Model file for the job. Use its own axes, mm. A direction names the side the tool comes from. Round coordinates to 2 decimals unless told otherwise and drop trailing zeros. Loops run counter-clockwise (first coordinate to the right, second up) from the corner with the lowest first, then second, coordinate; pieces in that order, holes last. Notation, with made-up numbers: M 79.5,-34.75 L 133.5,-34.75 A9 ccw 133.5,-19.75 Z; hole C 18,51 d9. An arc over 180 degrees is marked long. Use a Markdown table: item, result. Add a question column.
Q1. Mould opens along X. For faces 1 (the face through (-1.859, 1.797, 19.72)), 2 (the face through (-51, -41, 133.971)), 3 (the face through (5, 3, 20)) say: +X half, -X half, draft (parallel to the pull), parting line (faces both ways), or undercut.
Q2. Probe line 1 (Z direction, x = 5.5, y = 2.3); line 2 (Y direction, x = 2, z = 22); line 3 (X direction, y = 1, z = 10). List the from-to ranges inside material, lowest first. Write a range as from..to.
Q3. Tool access for faces 4 (the face through (-1, -25, 16)), 5 (the face through (-87.05, -41.056, 113.966)), 6 (the face through (-1, -9, 40)), 7 (the face through (-3, -23, 36)), 8 (the face through (0, -23, 36)): list every direction of +Z, -Z, +X, -X, +Y, -Y with a clear straight run to the whole face (end or side of a thin tool).
Q4. Cut at B-B (x = -54.5). Give the cut face in (y, z).
Q5. Pin check, flat tips, straight feed: pin 1 (3 mm diameter, centred on x = 5.5, z = 10, fed in from -Y); pin 2 (22 mm diameter, centred on y = -24.5, z = 51.5, fed in from +X); pin 3 (1.5 mm diameter, centred on x = -1, z = 16.5, fed in from -Y). Stop position of each tip, or through.
Q6. Cut at C-C (y = -8). Give the cut face in (x, z), plus the area to 3 significant figures.
Q7. Cut at A-A (z = 105). Give the cut face in (x, y), plus the area to 3 significant figures.
from build123d import *

# Parameters (mm, degrees)
SM_BASE_FLANGE_1_DEPTH           = 40
M3X0_5_1_D                       = 2.5
SKETCH_22_W                      = 3
SKETCH_22_H                      = 12
EXTRUDE_6_DEPTH                  = 12
SKETCH_23_W                      = 3
SKETCH_23_H                      = 67
EXTRUDE_7_DEPTH                  = 8
CHAMFER_1_SIZE                   = 10
CHAMFER_2_SIZE                   = 5
SM_EDGE_FLANGE_1_STRIP_CUT_DEPTH = 8
SM_EDGE_FLANGE_1_DEPTH           = 8
SM_EDGE_FLANGE_2_STRIP_CUT_DEPTH = 8
SM_EDGE_FLANGE_2_DEPTH           = 8
SM_EDGE_FLANGE_3_STRIP_CUT_DEPTH = 8
SM_EDGE_FLANGE_3_DEPTH           = 8


# Sheet-metal steps are written as plain solids
with BuildPart() as part:
    # 草圖3 → 基材-凸緣1 (new body)
    with BuildSketch(Plane.XY):
        with BuildLine():
            Line((10, 0), (1, 0))
            ThreePointArc((1, 0), (0.292893219, -0.292893219), (0, -1))
            Line((0, -1), (0, -25))
            Line((0, -25), (-3, -25))
            Line((-3, -25), (-3, -1))
            ThreePointArc((-3, -1), (-1.828427125, 1.828427125), (1, 3))
            Line((1, 3), (10, 3))
            Line((10, 3), (10, 0))
        make_face()
    extrude(amount=SM_BASE_FLANGE_1_DEPTH)

    # M3x0.5 螺紋孔1 (through all)
    with Locations(Plane(origin=(0, 3, 0), x_dir=(1, 0, 0), z_dir=(0, 1, 0))):
        with Locations((5.5, -30), (5.5, -10)):
            Hole(M3X0_5_1_D / 2)

    # 草圖22 → 填料-伸長6 (add)
    with BuildSketch(Plane.XZ.offset(25)):
        with Locations((-1.5, 34)):
            Rectangle(SKETCH_22_W, SKETCH_22_H)
    extrude(amount=EXTRUDE_6_DEPTH)

    # 草圖23 → 填料-伸長7 (add)
    with BuildSketch(Plane.XZ.offset(37)):
        with Locations((-1.5, 61.5)):
            Rectangle(SKETCH_23_W, SKETCH_23_H)
    extrude(amount=EXTRUDE_7_DEPTH)

    # 導角1
    chamfer_1_edges = [part.edges().sort_by_distance(p)[0] for p in [
        (-1.5, -37, 40),
        (-1.5, -45, 28),
    ]]
    chamfer(chamfer_1_edges, length=CHAMFER_1_SIZE)

    # 導角2
    chamfer_2_edges = [part.edges().sort_by_distance(p)[0] for p in [
        (-1.5, -25, 0),
    ]]
    chamfer(chamfer_2_edges, length=CHAMFER_2_SIZE)

    # 邊線-凸緣1 strip (across the edge) → 邊線-凸緣1 strip cut (cut)
    with BuildSketch(Plane(origin=(-3, -45, 95), x_dir=(-0.8660254037844416, 0, -0.49999999999999495), z_dir=(0, 1, 0))):
        Polygon((-9.464101615, 10.392304845), (-2.464101615, -1.732050808), (0.133974596, -0.232050808), (-6.866025404, 11.892304845), align=None)
    extrude(amount=SM_EDGE_FLANGE_1_STRIP_CUT_DEPTH, mode=Mode.SUBTRACT)

    # 邊線-凸緣1 section (across the edge) → 邊線-凸緣1 (add)
    with BuildSketch(Plane(origin=(-3, -45, 95), x_dir=(-0.8660254037844416, 0, -0.49999999999999495), z_dir=(0, 1, 0))):
        with BuildLine():
            Line((-3, 0.267949192), (-3, 45))
            Line((-3, 45), (0, 45))
            Line((0, 45), (0, 0.267949192))
            ThreePointArc((0, 0.267949192), (0.034074174, 0.009130147), (0.133974596, -0.232050808))
            Line((0.133974596, -0.232050808), (-2.464101615, -1.732050808))
            ThreePointArc((-2.464101615, -1.732050808), (-2.863703305, -0.767326988), (-3, 0.267949192))
        make_face()
    extrude(amount=SM_EDGE_FLANGE_1_DEPTH)

    # 邊線-凸緣2 strip (across the edge) → 邊線-凸緣2 strip cut (cut)
    with BuildSketch(Plane(origin=(-25.5, -45, 133.97114317), x_dir=(0, 0, -1), z_dir=(0, 1, 0))):
        Polygon((-13.124355653, 4.113248654), (-1, -2.886751346), (0.5, -0.288675135), (-11.624355653, 6.711324865), align=None)
    extrude(amount=SM_EDGE_FLANGE_2_STRIP_CUT_DEPTH, mode=Mode.SUBTRACT)

    # 邊線-凸緣2 section (across the edge) → 邊線-凸緣2 (add)
    with BuildSketch(Plane(origin=(-25.5, -45, 133.97114317), x_dir=(0, 0, -1), z_dir=(0, 1, 0))):
        with BuildLine():
            Line((-3, 0.577350269), (-3, 50))
            Line((-3, 50), (0, 50))
            Line((0, 50), (0, 0.577350269))
            ThreePointArc((0, 0.577350269), (0.133974596, 0.077350269), (0.5, -0.288675135))
            Line((0.5, -0.288675135), (-1, -2.886751346))
            ThreePointArc((-1, -2.886751346), (-2.464101615, -1.422649731), (-3, 0.577350269))
        make_face()
    extrude(amount=SM_EDGE_FLANGE_2_DEPTH)

    # 邊線-凸緣3 strip (across the edge) → 邊線-凸緣3 strip cut (cut)
    with BuildSketch(Plane(origin=(-75.5, -45, 133.97114317), x_dir=(0.8660254037844312, 0, -0.5000000000000132), z_dir=(0, 1, 0))):
        Polygon((-13.124355653, 4.113248654), (-1, -2.886751346), (0.5, -0.288675135), (-11.624355653, 6.711324865), align=None)
    extrude(amount=SM_EDGE_FLANGE_3_STRIP_CUT_DEPTH, mode=Mode.SUBTRACT)

    # 邊線-凸緣3 section (across the edge) → 邊線-凸緣3 (add)
    with BuildSketch(Plane(origin=(-75.5, -45, 133.97114317), x_dir=(0.8660254037844312, 0, -0.5000000000000132), z_dir=(0, 1, 0))):
        with BuildLine():
            Line((-3, 0.577350269), (-3, 45))
            Line((-3, 45), (0, 45))
            Line((0, 45), (0, 0.577350269))
            ThreePointArc((0, 0.577350269), (0.133974596, 0.077350269), (0.5, -0.288675135))
            Line((0.5, -0.288675135), (-1, -2.886751346))
            ThreePointArc((-1, -2.886751346), (-2.464101615, -1.422649731), (-3, 0.577350269))
        make_face()
    extrude(amount=SM_EDGE_FLANGE_3_DEPTH)


solid = part.part
Checked values:
| question | item | result |
|---|---|---|
| 1 | face 1 | -X half |
| 1 | face 2 | undercut |
| 1 | face 3 | draft |
| 2 | line 1 | z = 0..8.75, 11.25..28.75, 31.25..40 |
| 2 | line 2 | y = 0..3 |
| 2 | line 3 | x = -2.46..4.25, 6.75..10 |
| 3 | face 4 | -Z, +X, -X, -Y |
| 3 | face 5 | -Z, +Y, -Y |
| 3 | face 6 | +Z, +X, -X, +Y |
| 3 | face 7 | -Z, -X, +Y, -Y |
| 3 | face 8 | +Z, -Z, +X, -Y |
| 4 | outline | M -45,133.97 L -37,133.97 L -37,136.97 L -45,136.97 Z |
| 5 | pin 1 | stops at y = 0 |
| 5 | pin 2 | stops at x = 0 |
| 5 | pin 3 | stops at y = -25 |
| 6 | outline | M -3,0 L 0,0 L 0,40 L -3,40 Z |
| 6 | area | 120 mm^2 |
| 7 | outline | M -95.69,-45 L -92.23,-45 L -92.23,-37 L -95.69,-37 Z; M -8.77,-45 L -5.31,-45 L -5.31,-37 L -8.77,-37 Z |
| 7 | area | 55.4 mm^2 |
